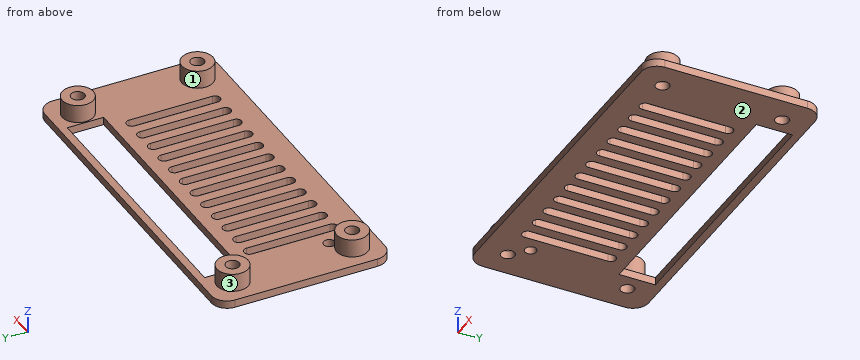
```python
from build123d import *

# Parameters (mm, degrees)
F0_R     = 3
F0_R_2   = 1.3
F1_DEPTH = 1.5
F2_DEPTH = 3.5
F3_W     = 51.5
F3_H     = 7
F4_DEPTH = 25
F5_R     = 1.1
F6_DEPTH = 25


with BuildPart() as f1:
    # F0 (on Top) → F1 (new body)
    with BuildSketch(Plane.XY):
        with BuildLine():
            Line((31.2, 16.7), (-31.2, 16.7))
            ThreePointArc((-31.2, 16.7), (-33.32132, 15.82132), (-34.2, 13.7))
            Line((-34.2, 13.7), (-34.2, -13.7))
            ThreePointArc((-34.2, -13.7), (-33.32132, -15.82132), (-31.2, -16.7))
            Line((-31.2, -16.7), (31.2, -16.7))
            ThreePointArc((31.2, -16.7), (33.32132, -15.82132), (34.2, -13.7))
            Line((34.2, -13.7), (34.2, 13.7))
            ThreePointArc((34.2, 13.7), (33.32132, 15.82132), (31.2, 16.7))
        make_face()
        with BuildLine():
            ThreePointArc((-32.7, 12.2), (-31.82132, 14.32132), (-29.7, 15.2))
            Line((-29.7, 15.2), (29.7, 15.2))
            ThreePointArc((29.7, 15.2), (31.82132, 14.32132), (32.7, 12.2))
            Line((32.7, 12.2), (32.7, -12.2))
            ThreePointArc((32.7, -12.2), (31.82132, -14.32132), (29.7, -15.2))
            Line((29.7, -15.2), (-29.7, -15.2))
            ThreePointArc((-29.7, -15.2), (-31.82132, -14.32132), (-32.7, -12.2))
            Line((-32.7, -12.2), (-32.7, 12.2))
        make_face(mode=Mode.SUBTRACT)
        with BuildLine():
            Line((29.7, 15.2), (-29.7, 15.2))
            ThreePointArc((-29.7, 15.2), (-31.82132, 14.32132), (-32.7, 12.2))
            Line((-32.7, 12.2), (-32.7, -12.2))
            ThreePointArc((-32.7, -12.2), (-31.82132, -14.32132), (-29.7, -15.2))
            Line((-29.7, -15.2), (29.7, -15.2))
            ThreePointArc((29.7, -15.2), (31.82132, -14.32132), (32.7, -12.2))
            Line((32.7, -12.2), (32.7, 12.2))
            ThreePointArc((32.7, 12.2), (31.82132, 14.32132), (29.7, 15.2))
        make_face()
        with Locations((-29, -11.5)):
            Circle(F0_R, mode=Mode.SUBTRACT)
        with Locations((29, -11.5)):
            Circle(F0_R, mode=Mode.SUBTRACT)
        with Locations((-29, 11.5)):
            Circle(F0_R, mode=Mode.SUBTRACT)
        with Locations((29, 11.5)):
            Circle(F0_R, mode=Mode.SUBTRACT)
        with Locations((-29, 11.5)):
            Circle(F0_R)
        with Locations((-29, 11.5)):
            Circle(F0_R_2, mode=Mode.SUBTRACT)
        with Locations((-29, -11.5)):
            Circle(F0_R)
        with Locations((-29, -11.5)):
            Circle(F0_R_2, mode=Mode.SUBTRACT)
        with Locations((29, -11.5)):
            Circle(F0_R)
        with Locations((29, -11.5)):
            Circle(F0_R_2, mode=Mode.SUBTRACT)
        with Locations((29, 11.5)):
            Circle(F0_R)
        with Locations((29, 11.5)):
            Circle(F0_R_2, mode=Mode.SUBTRACT)
    extrude(amount=-F1_DEPTH)

    # F0 (on Top) → F2 (join)
    with BuildSketch(Plane.XY):
        with Locations((-29, 11.5)):
            Circle(F0_R)
        with Locations((-29, 11.5)):
            Circle(F0_R_2, mode=Mode.SUBTRACT)
        with Locations((-29, -11.5)):
            Circle(F0_R)
        with Locations((-29, -11.5)):
            Circle(F0_R_2, mode=Mode.SUBTRACT)
        with Locations((29, -11.5)):
            Circle(F0_R)
        with Locations((29, -11.5)):
            Circle(F0_R_2, mode=Mode.SUBTRACT)
        with Locations((29, 11.5)):
            Circle(F0_R)
        with Locations((29, 11.5)):
            Circle(F0_R_2, mode=Mode.SUBTRACT)
    extrude(amount=F2_DEPTH)

    # F3 (on face) → F4 (cut)
    with BuildSketch(Plane(origin=(0, 0, -1.5), x_dir=(1, 0, 0), z_dir=(0, 0, -1))):
        with Locations((0, -11.7)):
            Rectangle(F3_W, F3_H)
        with BuildLine():
            ThreePointArc((-22, 12.3), (-22.707107, 12.007107), (-23, 11.3))
            Line((-23, 11.3), (-23, -4.7))
            ThreePointArc((-23, -4.7), (-22.707107, -5.407107), (-22, -5.7))
            ThreePointArc((-22, -5.7), (-21.292893, -5.407107), (-21, -4.7))
            Line((-21, -4.7), (-21, 11.3))
            ThreePointArc((-21, 11.3), (-21.292893, 12.007107), (-22, 12.3))
        make_face()
        with BuildLine():
            ThreePointArc((-18, 12.3), (-18.707107, 12.007107), (-19, 11.3))
            Line((-19, 11.3), (-19, -4.7))
            ThreePointArc((-19, -4.7), (-18.707107, -5.407107), (-18, -5.7))
            ThreePointArc((-18, -5.7), (-17.292893, -5.407107), (-17, -4.7))
            Line((-17, -4.7), (-17, 11.3))
            ThreePointArc((-17, 11.3), (-17.292893, 12.007107), (-18, 12.3))
        make_face()
        with BuildLine():
            ThreePointArc((-14, 12.3), (-14.707107, 12.007107), (-15, 11.3))
            Line((-15, 11.3), (-15, -4.7))
            ThreePointArc((-15, -4.7), (-14.707107, -5.407107), (-14, -5.7))
            ThreePointArc((-14, -5.7), (-13.292893, -5.407107), (-13, -4.7))
            Line((-13, -4.7), (-13, 11.3))
            ThreePointArc((-13, 11.3), (-13.292893, 12.007107), (-14, 12.3))
        make_face()
        with BuildLine():
            ThreePointArc((-10, 12.3), (-10.707107, 12.007107), (-11, 11.3))
            Line((-11, 11.3), (-11, -4.7))
            ThreePointArc((-11, -4.7), (-10.707107, -5.407107), (-10, -5.7))
            ThreePointArc((-10, -5.7), (-9.292893, -5.407107), (-9, -4.7))
            Line((-9, -4.7), (-9, 11.3))
            ThreePointArc((-9, 11.3), (-9.292893, 12.007107), (-10, 12.3))
        make_face()
        with BuildLine():
            ThreePointArc((-6, 12.3), (-6.707107, 12.007107), (-7, 11.3))
            Line((-7, 11.3), (-7, -4.7))
            ThreePointArc((-7, -4.7), (-6.707107, -5.407107), (-6, -5.7))
            ThreePointArc((-6, -5.7), (-5.292893, -5.407107), (-5, -4.7))
            Line((-5, -4.7), (-5, 11.3))
            ThreePointArc((-5, 11.3), (-5.292893, 12.007107), (-6, 12.3))
        make_face()
        with BuildLine():
            ThreePointArc((-2, 12.3), (-2.707107, 12.007107), (-3, 11.3))
            Line((-3, 11.3), (-3, -4.7))
            ThreePointArc((-3, -4.7), (-2.707107, -5.407107), (-2, -5.7))
            ThreePointArc((-2, -5.7), (-1.292893, -5.407107), (-1, -4.7))
            Line((-1, -4.7), (-1, 11.3))
            ThreePointArc((-1, 11.3), (-1.292893, 12.007107), (-2, 12.3))
        make_face()
        with BuildLine():
            ThreePointArc((2, 12.3), (1.292893, 12.007107), (1, 11.3))
            Line((1, 11.3), (1, -4.7))
            ThreePointArc((1, -4.7), (1.292893, -5.407107), (2, -5.7))
            ThreePointArc((2, -5.7), (2.707107, -5.407107), (3, -4.7))
            Line((3, -4.7), (3, 11.3))
            ThreePointArc((3, 11.3), (2.707107, 12.007107), (2, 12.3))
        make_face()
        with BuildLine():
            ThreePointArc((6, 12.3), (5.292893, 12.007107), (5, 11.3))
            Line((5, 11.3), (5, -4.7))
            ThreePointArc((5, -4.7), (5.292893, -5.407107), (6, -5.7))
            ThreePointArc((6, -5.7), (6.707107, -5.407107), (7, -4.7))
            Line((7, -4.7), (7, 11.3))
            ThreePointArc((7, 11.3), (6.707107, 12.007107), (6, 12.3))
        make_face()
        with BuildLine():
            ThreePointArc((10, 12.3), (9.292893, 12.007107), (9, 11.3))
            Line((9, 11.3), (9, -4.7))
            ThreePointArc((9, -4.7), (9.292893, -5.407107), (10, -5.7))
            ThreePointArc((10, -5.7), (10.707107, -5.407107), (11, -4.7))
            Line((11, -4.7), (11, 11.3))
            ThreePointArc((11, 11.3), (10.707107, 12.007107), (10, 12.3))
        make_face()
        with BuildLine():
            ThreePointArc((14, 12.3), (13.292893, 12.007107), (13, 11.3))
            Line((13, 11.3), (13, -4.7))
            ThreePointArc((13, -4.7), (13.292893, -5.407107), (14, -5.7))
            ThreePointArc((14, -5.7), (14.707107, -5.407107), (15, -4.7))
            Line((15, -4.7), (15, 11.3))
            ThreePointArc((15, 11.3), (14.707107, 12.007107), (14, 12.3))
        make_face()
        with BuildLine():
            ThreePointArc((18, 12.3), (17.292893, 12.007107), (17, 11.3))
            Line((17, 11.3), (17, -4.7))
            ThreePointArc((17, -4.7), (17.292893, -5.407107), (18, -5.7))
            ThreePointArc((18, -5.7), (18.707107, -5.407107), (19, -4.7))
            Line((19, -4.7), (19, 11.3))
            ThreePointArc((19, 11.3), (18.707107, 12.007107), (18, 12.3))
        make_face()
        with BuildLine():
            ThreePointArc((22, 12.3), (21.292893, 12.007107), (21, 11.3))
            Line((21, 11.3), (21, -4.7))
            ThreePointArc((21, -4.7), (21.292893, -5.407107), (22, -5.7))
            ThreePointArc((22, -5.7), (22.707107, -5.407107), (23, -4.7))
            Line((23, -4.7), (23, 11.3))
            ThreePointArc((23, 11.3), (22.707107, 12.007107), (22, 12.3))
        make_face()
    extrude(amount=-F4_DEPTH, mode=Mode.SUBTRACT)

    # F5 (on face) → F6 (cut)
    with BuildSketch(Plane(origin=(0, 0, -1.5), x_dir=(1, 0, 0), z_dir=(0, 0, -1))):
        with Locations((-26.100862, 8.600862)):
            Circle(F5_R)
    extrude(amount=-F6_DEPTH, mode=Mode.SUBTRACT)


solid = f1.part
```
Model file for the job. Use its own axes, mm. Face numbers are marked on the shaded views. Coordinates: 2 decimals unless noted, no trailing zeros. Loops run counter-clockwise (first coordinate to the right, second up) from the corner with the lowest first, then second, coordinate; pieces in that order, holes last. Notation, with made-up numbers: (15.5, 32.5) - (31.5, 32.5) arc R32 cw to (31.5, 58.5) - close; hole circle Ø10 at (-8, 81.25). An arc over 180 degrees is marked (long way). Answer as a JSON object with one key per item and string values. Group by question number.
(1) Cut at B-B (x = 29). Give the cut face in (y, z).
(2) Flat gauge pin, fed straight in: pin 1 (6 mm diameter, centred on x = -16.5, y = -0.5, fed in from +Z). Where does the tip first touch, or does it go through?
(3) Cut at C-C (y = 11.5). Give the cut face in (x, z).
(4) Cut at D-D (y = 0). State how many separate pieces and enclosed holes the cut face has, then the cut area to 3 significant figures.
(5) Two-plate mould, pull along X, no slides. Class the marked faces 1, 2 and 3: released by +X, released by -X, zero draft, split by the parting line, or undercut.
(6) Probe line 1 along Y through (x, z) = (-29, 1.3); line 2 along Y through (x, z) = (-29, -1.05); line 3 along Y through (x, z) = (-14, -0.35). List the from-to ranges inside material, lowest first.
(7) Cut at A-A (z = 0.9). Give the cut face in (x, y).
Geometry says:
{
 "1": {"outline": "(-16.7, -1.5) - (-12.8, -1.5) - (-12.8, 3.5) - (-14.5, 3.5) - (-14.5, 0) - (-16.7, 0) - close; (-10.2, -1.5) - (10.2, -1.5) - (10.2, 3.5) - (8.5, 3.5) - (8.5, 0) - (-8.5, 0) - (-8.5, 3.5) - (-10.2, 3.5) - close; (12.8, -1.5) - (16.7, -1.5) - (16.7, 0) - (14.5, 0) - (14.5, 3.5) - (12.8, 3.5) - close"},
 "2": {"pin 1": "stops at z = 0"},
 "3": {"outline": "(-34.2, -1.5) - (-30.3, -1.5) - (-30.3, 3.5) - (-32, 3.5) - (-32, 0) - (-34.2, 0) - close; (-27.7, -1.5) - (-25.75, -1.5) - (-25.75, 0) - (-26, 0) - (-26, 3.5) - (-27.7, 3.5) - close; (25.75, -1.5) - (27.7, -1.5) - (27.7, 3.5) - (26, 3.5) - (26, 0) - (25.75, 0) - close; (30.3, -1.5) - (34.2, -1.5) - (34.2, 0) - (32, 0) - (32, 3.5) - (30.3, 3.5) - close"},
 "4": {"separate pieces": "13", "enclosed holes": "0", "area": "66.6 mm^2"},
 "5": {"face 1": "undercut", "face 2": "zero draft", "face 3": "undercut"},
 "6": {"line 1": "y = -14.5 to -12.8, -10.2 to -8.5, 8.5 to 10.2, 12.8 to 14.5", "line 2": "y = -16.7 to -12.8, -10.2 to 10.2, 12.8 to 16.7", "line 3": "y = -16.7 to -12.3, 5.7 to 8.2, 15.2 to 16.7"},
 "7": {"outline": "circle Ø6 at (-29, -11.5); circle Ø6 at (-29, 11.5); circle Ø6 at (29, -11.5); circle Ø6 at (29, 11.5); hole circle Ø2.6 at (-29, -11.5); hole circle Ø2.6 at (-29, 11.5); hole circle Ø2.6 at (29, -11.5); hole circle Ø2.6 at (29, 11.5)"}
}
